Check sheet for the modelled part. Datum: model origin and axes. Units: mm. A direction names the side the tool comes from. Coordinates: 2 decimals unless noted, no trailing zeros. Loops run counter-clockwise (first coordinate to the right, second up) from the corner with the lowest first, then second, coordinate; pieces in that order, holes last. Notation, with made-up numbers: (17.5, -10.75) -> (45.5, -10.75) arc R9 cw to (45.5, 6.25) -> close; hole circle Ø6 at (48, 31). An arc over 180 degrees is marked (long way). Use one line per item in the form item = value.
from build123d import *

# Parameters (mm, degrees)
F0_R            = 78.299536584
F0_R_2          = 58.8964149972
F1_DEPTH        = 25.4
F2_W            = 24.3125222623
F2_H            = 12.9293575883
F3_DEPTH        = 90.7285287976
F3_COPIES_COUNT = 5


# Not quite as in the source:
# - a pattern or mirror of a feature is missing from the dataset's text; its kind, count and spacing are read off the source's solid


with BuildPart() as f1:
    # F0 (on Top) → F1 (new body)
    with BuildSketch(Plane.XY):
        Circle(F0_R)
        Circle(F0_R_2, mode=Mode.SUBTRACT)
    extrude(amount=F1_DEPTH)

    # F2 (on Front) → F3 (join)
    with BuildSketch(Plane.XZ):
        with Locations((0, 16.8866589665)):
            Rectangle(F2_W, F2_H)
    f3 = extrude(amount=F3_DEPTH)

    # F3_copies: F3 ×5 about axis
    f3_copies_axis = Axis((0, 0, 0), (0, 0, 1))
    for i in range(1, F3_COPIES_COUNT):
        add(f3.rotate(f3_copies_axis, i * 360 / F3_COPIES_COUNT))


solid = f1.part
(1) Section check B-B, the plane y = 0. Record the boundary of the cut face in (x, z), plus the area to 3 significant figures.
Established:
outline = (-78.3, 0) -> (-58.9, 0) -> (-58.9, 25.4) -> (-78.3, 25.4) -> close; (-39.34, 10.42) -> (39.34, 10.42) -> (39.34, 23.35) -> (-39.34, 23.35) -> close; (58.9, 0) -> (78.3, 0) -> (78.3, 25.4) -> (58.9, 25.4) -> close
area = 2,000 mm²
(2) Mould release check, pull along Y, two halves, no side actions. Record for faces 1 (the flat face through (-31.33, -22.96, 16.8)), 2 (the flat face through (80, -26, 10.422)), 3 (the flat face through (76.08, -37.5, 16.8)): +Y half, -Y half, draft (parallel to the pull), parting line (faces both ways), or undercut.
Established:
face_1 = undercut
face_2 = draft
face_3 = -Y half
(3) Go/stop test with flat-tipped pins: P1, Ø5, axis at y = -24.5, z = 16, coming from the -X side; P2, Ø12, axis at x = 39, z = 15, coming from the -Y side; P3, Ø6, axis at x = 84, y = -24, coming from the +Z side; P4, Ø7.5, axis at x = -44, y = 68, coming from the -Z side. Record where each tip stops, or that it passes through.
Established:
P1 = -88.25
P2 = -71.01
P3 = 23.35
P4 = 0
(4) Section check A-A, the plane y = 33. Record the boundary of the cut face in (x, z), plus the area to 3 significant figures.
Established:
outline = (-71.01, 0) -> (-48.78, 0) -> (-48.78, 25.4) -> (-71.01, 25.4) -> close; (-39, 10.42) -> (-8.95, 10.42) -> (-8.95, 23.35) -> (-39, 23.35) -> close; (8.95, 10.42) -> (39, 10.42) -> (39, 23.35) -> (8.95, 23.35) -> close; (48.78, 0) -> (71.01, 0) -> (71.01, 25.4) -> (48.78, 25.4) -> close
area = 1,910 mm²
(5) Section check C-C, the plane z = 3.25. Record the boundary of the cut face in (x, y).
Established:
outline = circle Ø156.6 at (0, 0); hole circle Ø117.79 at (0, 0)
(6) Scan lines: line 1 along Y through (x, z) = (0, 7.75); line 2 along Y through (x, z) = (38.5, 10.5); line 3 along Y through (x, z) = (8.5, 16.25). Record each from-to range of solid material in increasing order.
Established:
line_1 = -78.3 to -58.9, 58.9 to 78.3
line_2 = -68.18 to -44.57, -25.29 to 0.27, 32.31 to 73.67
line_3 = -90.73 to 32.38, 58.28 to 77.84
(7) Section check D-D, the plane y = -52. Record the boundary of the cut face in (x, z), plus the area to 3 significant figures.
Established:
outline = (-58.54, 0) -> (-27.65, 0) -> (-27.65, 25.4) -> (-58.54, 25.4) -> close; (-12.16, 10.42) -> (12.16, 10.42) -> (12.16, 23.35) -> (-12.16, 23.35) -> close; (27.65, 0) -> (58.54, 0) -> (58.54, 25.4) -> (27.65, 25.4) -> close
area = 1,880 mm²
(8) Tool access check on faces 4 (the flat face through (-31.52, 22.7, 16.8)), 5 (the flat face through (-76.08, -37.5, 16.8)), 6 (the flat face through (49, 68, 10.422)). Record the directions out of +Z, -Z, +X, -X, +Y, -Y that give a thin tool (end or side, any length) a straight path to the whole face; none if there is none.
Established:
face_4 = +Z, -Z
face_5 = +Z, -Z, -Y
face_6 = -Z, +X, +Y
